For this review, take the finished solid that the model builds, in its own axes (mm). Face numbers are marked on the shaded views. A direction names the side the tool comes from. Coordinates: 2 decimals unless noted, no trailing zeros. Loops run counter-clockwise (first coordinate to the right, second up) from the corner with the lowest first, then second, coordinate; pieces in that order, holes last. Notation, with made-up numbers: M 5.25,52.25 L 41.25,52.25 A20 cw 41.25,82.25 Z; hole C -30,56.5 d8. An arc over 180 degrees is marked long. Write item = value, one per line.
from build123d import *

# Parameters (mm, degrees)
SKIZZE1_W                       = 44.1
SKIZZE1_H                       = 33
AUFSATZ_LINEAR_AUSTRAGEN1_DEPTH = 3
SKIZZE2_W                       = 3
SKIZZE2_H                       = 33
AUFSATZ_LINEAR_AUSTRAGEN2_DEPTH = 24
SKIZZE3_W                       = 33
SKIZZE3_H                       = 12
SCHNITT_LINEAR_AUSTRAGEN1_DEPTH = 24
SKIZZE4_R                       = 1.2
SCHNITT_LINEAR_AUSTRAGEN2_DEPTH = 10
SKIZZE5_R                       = 1.05
SCHNITT_LINEAR_AUSTRAGEN3_DEPTH = 10
SKIZZE6_R                       = 3.5
SCHNITT_LINEAR_AUSTRAGEN4_DEPTH = 10


with BuildPart() as part:
    # Skizze1 → Aufsatz-Linear austragen1 (new body)
    with BuildSketch(Plane(origin=(0, 0, 0), x_dir=(1, 0, 0), z_dir=(0, 1, 0))):
        Rectangle(SKIZZE1_W, SKIZZE1_H)
    extrude(amount=AUFSATZ_LINEAR_AUSTRAGEN1_DEPTH)

    # Skizze2 → Aufsatz-Linear austragen2 (add)
    with BuildSketch(Plane(origin=(0, 3, 0), x_dir=(1, 0, 0), z_dir=(0, 1, 0))):
        with Locations((-20.55, 0)):
            Rectangle(SKIZZE2_W, SKIZZE2_H)
        with Locations((20.55, 0)):
            Rectangle(SKIZZE2_W, SKIZZE2_H)
    extrude(amount=AUFSATZ_LINEAR_AUSTRAGEN2_DEPTH)

    # Skizze3 → Schnitt-Linear austragen1 (cut)
    with BuildSketch(Plane(origin=(22.05, 0, 0), x_dir=(0, 0, -1), z_dir=(1, 0, 0))):
        with Locations((0, 21)):
            Rectangle(SKIZZE3_W, SKIZZE3_H)
    extrude(amount=-SCHNITT_LINEAR_AUSTRAGEN1_DEPTH, mode=Mode.SUBTRACT)

    # Skizze4 → Schnitt-Linear austragen2 (cut)
    with BuildSketch(Plane(origin=(-19.05, 0, 0), x_dir=(0, 0, -1), z_dir=(1, 0, 0))):
        with Locations((-5.7, 20.85)):
            Circle(SKIZZE4_R)
    extrude(amount=-SCHNITT_LINEAR_AUSTRAGEN2_DEPTH, mode=Mode.SUBTRACT)

    # Skizze5 → Schnitt-Linear austragen3 (cut)
    with BuildSketch(Plane(origin=(22.05, 0, 0), x_dir=(0, 0, -1), z_dir=(1, 0, 0))):
        with Locations((-5.3, 10.5)):
            Circle(SKIZZE5_R)
        with Locations((-5.3, 6.5)):
            Circle(SKIZZE5_R)
    extrude(amount=-SCHNITT_LINEAR_AUSTRAGEN3_DEPTH, mode=Mode.SUBTRACT)

    # Skizze6 → Schnitt-Linear austragen4 (cut)
    with BuildSketch(Plane.XZ):
        with Locations(Location((-12, 0, 0), (0, 0, 270))):
            Circle(SKIZZE6_R)
        with Locations(Location((0, -11.5, 0), (0, 0, 270))):
            Circle(SKIZZE6_R)
        with Locations(Location((12, 0, 0), (0, 0, 270))):
            Circle(SKIZZE6_R)
        with Locations(Location((0, 11.5, 0), (0, 0, 270))):
            Circle(SKIZZE6_R)
    extrude(amount=-SCHNITT_LINEAR_AUSTRAGEN4_DEPTH, mode=Mode.SUBTRACT)


solid = part.part
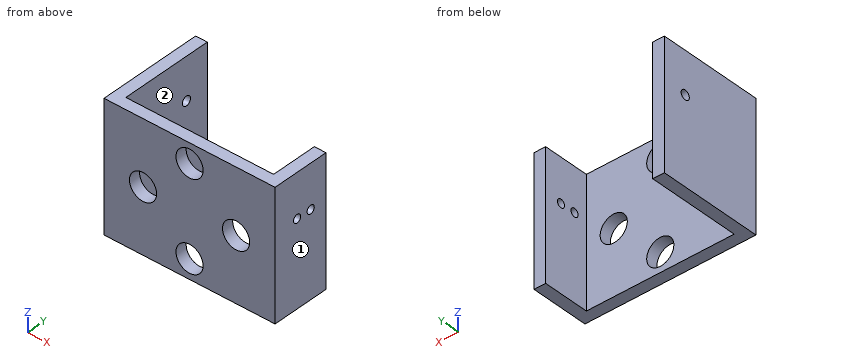
Q1. For pin 1 Ø2.5 at (x, z) = (20.5, 2) entering from +Y; pin 2 Ø10 at (x, z) = (-16, -12.5) entering from +Y; pin 3 Ø2 at (x, z) = (4.5, 7) entering from +Y, all flat-tipped, find the tip position at first contact; note any pin that passes through.
Solved:
pin_1 = 15
pin_2 = 27
pin_3 = 3
Q2. Add section D-D (x = 0). Write out the cut boundary in (y, z).
Solved:
outline = M 0,-16.5 L 3,-16.5 L 3,-15 L 0,-15 Z; M 0,-8 L 3,-8 L 3,8 L 0,8 Z; M 0,15 L 3,15 L 3,16.5 L 0,16.5 Z
Q3. For line 1 along X through (y, z) = (0.8, 11.5); line 2 along Y through (x, z) = (20, 5); line 3 along Y through (x, z) = (-8, 11.5), list the stretches that pass through material, from the lowest coordinate up.
Solved:
line_1 = -22.05 to -3.5, 3.5 to 22.05
line_2 = 0 to 5.49, 7.51 to 9.49, 11.51 to 15
line_3 = 0 to 3
Q4. Machinability: for the marked faces 1 and 2, which of the approach directions +Z, -Z, +X, -X, +Y, -Y give a long, thin tool a straight path to every point of the face, cutting with its end or side? Answer none if there is none.
Solved:
face_1 = +Z, -Z, +X, +Y, -Y
face_2 = +Z, -Z, +Y
Q5. Add section A-A (z = 0). Write out the cut boundary in (x, y).
Solved:
outline = M -22.05,0 L -15.5,0 L -15.5,3 L -19.05,3 L -19.05,27 L -22.05,27 Z; M -8.5,0 L 8.5,0 L 8.5,3 L -8.5,3 Z; M 15.5,0 L 22.05,0 L 22.05,15 L 19.05,15 L 19.05,3 L 15.5,3 Z
Q6. Add section C-C (y = 8.75). Write out the cut boundary in (x, z).
Solved:
outline = M -22.05,-16.5 L -19.05,-16.5 L -19.05,16.5 L -22.05,16.5 Z; M 19.05,-16.5 L 22.05,-16.5 L 22.05,16.5 L 19.05,16.5 Z
Q7. Add section B-B (z = -11.5). Write out the cut boundary in (x, y).
Solved:
outline = M -22.05,0 L -3.5,0 L -3.5,3 L -19.05,3 L -19.05,27 L -22.05,27 Z; M 3.5,0 L 22.05,0 L 22.05,15 L 19.05,15 L 19.05,3 L 3.5,3 Z
